Geometry: final body of the model. Coordinates: model frame, mm. Face numbers are marked on the shaded views. A direction names the side the tool comes from. Give positions to 0.01 mm unless a question says otherwise; leave off trailing zeros. Write each loop counter-clockwise with the first axis right and the second up, starting at its lowest first coordinate (ties: lowest second). Pieces come first, ordered by that corner, then holes.
Q1. Line query: L1, parallel to Y at x = 0, z = 24.75; L2, parallel to X at y = 1, z = 17; L3, parallel to Z at x = 9.5, y = 6. Output: solid intervals per line, ascending.
Q2. Cut plane C-C on z = 4.75. Return the cut outline in (x, y) (1 decimal).
Q3. Cut plane A-A on z = 10.75. Return the cut outline in (x, y) (1 decimal).
Q4. Draft query along X for the marked faces 3, 4 and 5. Return one class per face: pulls with the +X half, pulls with the -X half, needs draft (parallel to the pull), parting line crosses it, or undercut.
Q5. Cut plane B-B on x = 0. Return the cut outline in (y, z), plus the area to 3 significant figures.
Q6. Reachability of the marked faces 1 and 2 from +Z, -Z, +X, -X, +Y, -Y: full face, straight path, thin tool, end or side. Return the list, or none.
Q7. Pin query (flat end, axial travel): pin 1 (3 mm diameter, centred on y = 4, z = 6.5, fed in from -X); pin 2 (6 mm diameter, centred on x = 9, z = 4, fed in from +Y); pin 3 (3 mm diameter, centred on x = 1, z = 26, fed in from +Y). Return the tip coordinate at first contact, or that it passes through.
Q8. Cut plane D-D on z = 24.25. Return the cut outline in (x, y) (3 decimals).
```python
from build123d import *

# Parameters (mm, degrees)
F1_R      = 9
F2_DEPTH  = 12
F2_FACE_R = 9
F3_DEPTH  = 18
F5_DEPTH  = 12
F6_SIZE   = 1.99999


# Not quite as in the source:
# - a fillet or chamfer is up to 0.001 mm smaller than in the source, because OpenCascade refuses the exact size


with BuildPart() as f2:
    # F1 (on Top) → F2 (new body)
    with BuildSketch(Plane.XY):
        Circle(F1_R)
        with BuildLine():
            ThreePointArc((-3.5524069735, -1.2012096798), (-0.6086763711, 3.7002720272), (3.75, 0))
            ThreePointArc((3.75, 0), (3.7002720272, -0.6086763711), (3.5524069735, -1.2012096798))
            ThreePointArc((3.5524069735, -1.2012096798), (3.7247345197, -1.339079143), (3.7896742158, -1.55))
            ThreePointArc((3.7896742158, -1.55), (3.6098282416, -1.8702185288), (3.242794716, -1.8832903202))
            ThreePointArc((3.242794716, -1.8832903202), (0, -3.75), (-3.242794716, -1.8832903202))
            ThreePointArc((-3.242794716, -1.8832903202), (-3.7561416374, -1.705), (-3.5524069735, -1.2012096798))
        make_face(mode=Mode.SUBTRACT)
        with BuildLine():
            Line((3.0396742158, -1.55), (-3.0396742158, -1.55))
            ThreePointArc((-3.0396742158, -1.55), (-3.0944556869, -1.7451540258), (-3.242794716, -1.8832903202))
            ThreePointArc((-3.242794716, -1.8832903202), (0, -3.75), (3.242794716, -1.8832903202))
            ThreePointArc((3.242794716, -1.8832903202), (3.0944556869, -1.7451540258), (3.0396742158, -1.55))
        make_face()
    extrude(amount=F2_DEPTH)

    # F1 (on Top) + F2_face (on face) → F3 (join)
    with BuildSketch(Plane.XY):
        with BuildLine():
            ThreePointArc((-4.2766728371, 14.4583333333), (-5.2456206791, 14.8589384831), (-6.2840906994, 14.7142857143))
            ThreePointArc((-6.2840906994, 14.7142857143), (-9.4045640367, 12.94427191), (-12.0522264909, 10.5234897545))
            ThreePointArc((-12.0522264909, 10.5234897545), (-12.5107043337, 9.5805462385), (-12.4291275454, 8.5352282801))
            ThreePointArc((-12.4291275454, 8.5352282801), (-12.3637347118, 4.0172209269), (-15.0722567175, 0.4005131406))
            ThreePointArc((-15.0722567175, 0.4005131406), (-15.7526762055, -0.3972172192), (-15.9360081315, -1.4295610629))
            ThreePointArc((-15.9360081315, -1.4295610629), (-15.2169042607, -4.94427191), (-13.7327763109, -8.2104113658))
            ThreePointArc((-13.7327763109, -8.2104113658), (-12.9776611805, -8.9378352769), (-11.9582961107, -9.1832721545))
            ThreePointArc((-11.9582961107, -9.1832721545), (-7.6412082798, -10.5172209269), (-5.0384941015, -14.2108025995))
            ThreePointArc((-5.0384941015, -14.2108025995), (-4.4900686296, -15.1044322255), (-3.5649039709, -15.5978030401))
            ThreePointArc((-3.5649039709, -15.5978030401), (0, -16), (3.5649039709, -15.5978030401))
            ThreePointArc((3.5649039709, -15.5978030401), (4.4900686296, -15.1044322255), (5.0384941015, -14.2108025995))
            ThreePointArc((5.0384941015, -14.2108025995), (7.6412082798, -10.5172209269), (11.9582961107, -9.1832721545))
            ThreePointArc((11.9582961107, -9.1832721545), (12.9776611805, -8.9378352769), (13.7327763109, -8.2104113658))
            ThreePointArc((13.7327763109, -8.2104113658), (15.2169042607, -4.94427191), (15.9360081315, -1.4295610629))
            ThreePointArc((15.9360081315, -1.4295610629), (15.7526762055, -0.3972172192), (15.0722567175, 0.4005131406))
            ThreePointArc((15.0722567175, 0.4005131406), (12.3637347118, 4.0172209269), (12.4291275454, 8.5352282801))
            ThreePointArc((12.4291275454, 8.5352282801), (12.5107043337, 9.5805462385), (12.0522264909, 10.5234897545))
            ThreePointArc((12.0522264909, 10.5234897545), (9.4045640367, 12.94427191), (6.2840906994, 14.7142857143))
            ThreePointArc((6.2840906994, 14.7142857143), (5.2456206791, 14.8589384831), (4.2766728371, 14.4583333333))
            ThreePointArc((4.2766728371, 14.4583333333), (0, 13), (-4.2766728371, 14.4583333333))
        make_face()
        Circle(F1_R, mode=Mode.SUBTRACT)
        with BuildLine():
            ThreePointArc((3.5524069735, -1.2012096798), (3.7002720272, -0.6086763711), (3.75, 0))
            ThreePointArc((3.75, 0), (-0.6086763711, 3.7002720272), (-3.5524069735, -1.2012096798))
            ThreePointArc((-3.5524069735, -1.2012096798), (-3.2037533587, -1.2399396961), (-3.0396742158, -1.55))
            Line((-3.0396742158, -1.55), (3.0396742158, -1.55))
            ThreePointArc((3.0396742158, -1.55), (3.2037533587, -1.2399396961), (3.5524069735, -1.2012096798))
        make_face()
        with BuildLine():
            ThreePointArc((-3.4146742158, -1.55), (-3.487903202, -1.3773275768), (-3.5524069735, -1.2012096798))
            ThreePointArc((-3.5524069735, -1.2012096798), (-3.7561416374, -1.705), (-3.242794716, -1.8832903202))
            ThreePointArc((-3.242794716, -1.8832903202), (-3.332903202, -1.7187949983), (-3.4146742158, -1.55))
        make_face()
        with BuildLine():
            ThreePointArc((-3.0396742158, -1.55), (-3.2037533587, -1.2399396961), (-3.5524069735, -1.2012096798))
            ThreePointArc((-3.5524069735, -1.2012096798), (-3.487903202, -1.3773275768), (-3.4146742158, -1.55))
            Line((-3.4146742158, -1.55), (-3.0396742158, -1.55))
        make_face()
        with BuildLine():
            Line((-3.0396742158, -1.55), (-3.4146742158, -1.55))
            ThreePointArc((-3.4146742158, -1.55), (-3.332903202, -1.7187949983), (-3.242794716, -1.8832903202))
            ThreePointArc((-3.242794716, -1.8832903202), (-3.0944556869, -1.7451540258), (-3.0396742158, -1.55))
        make_face()
        with BuildLine():
            ThreePointArc((3.4146742158, -1.55), (3.487903202, -1.3773275768), (3.5524069735, -1.2012096798))
            ThreePointArc((3.5524069735, -1.2012096798), (3.2037533587, -1.2399396961), (3.0396742158, -1.55))
            Line((3.0396742158, -1.55), (3.4146742158, -1.55))
        make_face()
        with BuildLine():
            ThreePointArc((3.242794716, -1.8832903202), (3.332903202, -1.7187949983), (3.4146742158, -1.55))
            Line((3.4146742158, -1.55), (3.0396742158, -1.55))
            ThreePointArc((3.0396742158, -1.55), (3.0944556869, -1.7451540258), (3.242794716, -1.8832903202))
        make_face()
        with BuildLine():
            ThreePointArc((3.7896742158, -1.55), (3.7247345197, -1.339079143), (3.5524069735, -1.2012096798))
            ThreePointArc((3.5524069735, -1.2012096798), (3.487903202, -1.3773275768), (3.4146742158, -1.55))
            ThreePointArc((3.4146742158, -1.55), (3.332903202, -1.7187949983), (3.242794716, -1.8832903202))
            ThreePointArc((3.242794716, -1.8832903202), (3.6098282416, -1.8702185288), (3.7896742158, -1.55))
        make_face()
    with BuildSketch(Plane(origin=(0, -0.1158950357, 12), x_dir=(1, 0, 0), z_dir=(0, 0, 1))):
        with Locations((0, 0.1158950357)):
            Circle(F2_FACE_R)
        with BuildLine():
            ThreePointArc((-3.5524069735, -1.0853146441), (0, 3.8658950357), (3.5524069735, -1.0853146441))
            ThreePointArc((3.5524069735, -1.0853146441), (3.6255950728, -1.7441652682), (3.0396742158, -1.4341049643))
            Line((3.0396742158, -1.4341049643), (-3.0396742158, -1.4341049643))
            ThreePointArc((-3.0396742158, -1.4341049643), (-3.6255950728, -1.7441652682), (-3.5524069735, -1.0853146441))
        make_face(mode=Mode.SUBTRACT)
    extrude(amount=F3_DEPTH)

    # F4 (on face) → F5 (cut)
    with BuildSketch(Plane.XY.offset(18)):
        with BuildLine():
            ThreePointArc((2.891366459, -0.8), (2.9727175595, -0.4036710437), (3, 0))
            ThreePointArc((3, 0), (-0.4036710437, 2.9727175595), (-2.891366459, -0.8))
            Line((-2.891366459, -0.8), (2.891366459, -0.8))
        make_face()
    extrude(amount=-F5_DEPTH, mode=Mode.SUBTRACT)

    # F6 (size 2 in the source; OpenCascade refuses exactly that, so slightly less here)
    f6_edges = [f2.edges().sort_by_distance(p)[0] for p in [
        (0, -16, 18),
        (0, -16, 0),
    ]]
    chamfer(f6_edges, length=F6_SIZE)


solid = f2.part
```
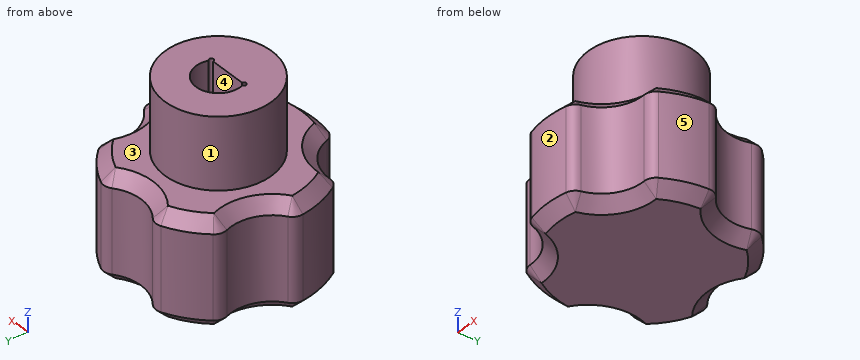
Data:
1. L1: y = -9 to -1.55, 3.75 to 9
1. L2: x = -12.92 to -2.83, 2.83 to 12.92
1. L3: z = 0 to 18
2. outline: (-15.9, -1.4) arc R16 ccw to (-13.7, -8.2) arc R2 ccw to (-12, -9.2) arc R7 cw to (-5, -14.2) arc R2 ccw to (-3.6, -15.6) arc R16 ccw to (3.6, -15.6) arc R2 ccw to (5, -14.2) arc R7 cw to (12, -9.2) arc R2 ccw to (13.7, -8.2) arc R16 ccw to (15.9, -1.4) arc R2 ccw to (15.1, 0.4) arc R7 cw to (12.4, 8.5) arc R2 ccw to (12.1, 10.5) arc R16 ccw to (6.3, 14.7) arc R2 ccw to (4.3, 14.5) arc R7 cw to (-4.3, 14.5) arc R2 ccw to (-6.3, 14.7) arc R16 ccw to (-12.1, 10.5) arc R2 ccw to (-12.4, 8.5) arc R7 cw to (-15.1, 0.4) arc R2 ccw to start
3. outline: (-15.9, -1.4) arc R16 ccw to (-13.7, -8.2) arc R2 ccw to (-12, -9.2) arc R7 cw to (-5, -14.2) arc R2 ccw to (-3.6, -15.6) arc R16 ccw to (3.6, -15.6) arc R2 ccw to (5, -14.2) arc R7 cw to (12, -9.2) arc R2 ccw to (13.7, -8.2) arc R16 ccw to (15.9, -1.4) arc R2 ccw to (15.1, 0.4) arc R7 cw to (12.4, 8.5) arc R2 ccw to (12.1, 10.5) arc R16 ccw to (6.3, 14.7) arc R2 ccw to (4.3, 14.5) arc R7 cw to (-4.3, 14.5) arc R2 ccw to (-6.3, 14.7) arc R16 ccw to (-12.1, 10.5) arc R2 ccw to (-12.4, 8.5) arc R7 cw to (-15.1, 0.4) arc R2 ccw to start; hole (-2.9, -0.8) - (2.9, -0.8) arc R3 ccw (long way) to start
4. face 3: needs draft
4. face 4: undercut
4. face 5: pulls with the +X half
5. outline: (-16, 2) - (-14, 0) - (11, 0) - (13, 2) - (13, 16) - (11, 18) - (9, 18) - (9, 30) - (3.75, 30) - (3.75, 18) - (3, 18) - (3, 6) - (-0.8, 6) - (-0.8, 18) - (-1.55, 18) - (-1.55, 30) - (-9, 30) - (-9, 18) - (-14, 18) - (-16, 16) - close
5. area: 621 mm2
6. face 1: +Z
6. face 2: +Z, -Z, -Y
7. pin 1: stops at x = -13.07
7. pin 2: stops at y = 14.81
7. pin 3: stops at y = 9
8. outline: circle Ø18 at (0, 0); hole (-3.552, -1.201) arc R0.375 ccw (long way) to (-3.04, -1.55) - (3.04, -1.55) arc R0.375 ccw (long way) to (3.552, -1.201) arc R3.75 ccw (long way) to start
